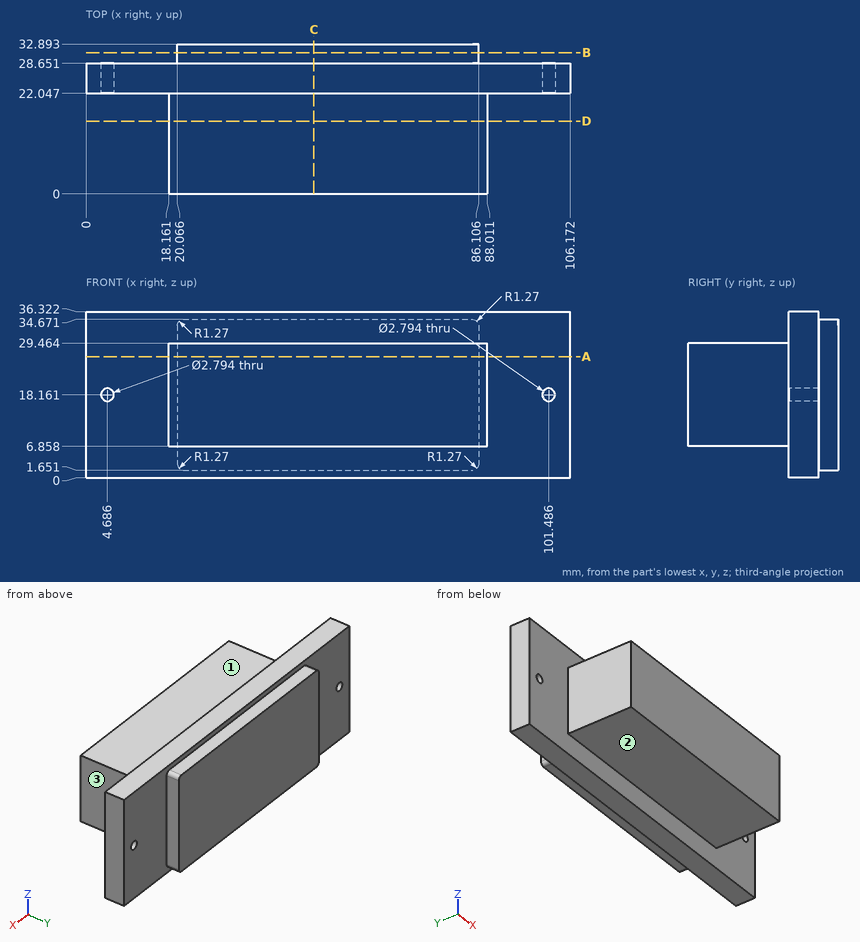
Design review of the part shown in the three views and the two pictorial views. Dimensions are in mm from the part's minimum x, y and z. A direction names the side the tool comes from. Round coordinates to 2 decimals unless told otherwise and drop trailing zeros. Loops run counter-clockwise (first coordinate to the right, second up) from the corner with the lowest first, then second, coordinate; pieces in that order, holes last. Notation, with made-up numbers: (45, 51) -> (58, 51) arc R30 ccw to (58, 90) -> close; hole circle Ø2 at (3.5, -17). An arc over 180 degrees is marked (long way). Answer as a JSON object with one key per item and string values. Group by question number.
1) We need section B-B on y = 31. Write out the cut boundary in (x, z).
2) We need section D-D on y = 16. Write out the cut boundary in (x, z), then the cut area to 3 significant figures.
3) For pin 1 Ø11 at (y, z) = (14, 15) entering from -X; pin 2 Ø6 at (x, y) = (73.5, 16.5) entering from -Z; pin 3 Ø1.3 at (x, y) = (55, 30.5) entering from -Z; pin 4 Ø1.7 at (x, z) = (4.69, 18.16) entering from -Y, all flat-tipped, find the tip position at first contact; note any pin that passes through.
4) For line 1 (X direction, y = 17, z = 22); line 2 (Z direction, x = 27, y = 31.5); line 3 (Y direction, x = 64.5, z = 33.5), list the stretches that pass through material, from the lowest coordinate up. Write a range as [from, to].
5) For the marked faces 1, 2 and 3, list the 3-axis set-ups (+Z, -Z, +X, -X, +Y, -Y) from which the entire face can be reached by the end or side of a thin tool; tool diameter is ignored.
6) We need section A-A on z = 26.5. Write out the cut boundary in (x, y), then the cut area to 3 significant figures.
7) We need section C-C on x = 50. Write out the cut boundary in (y, z), then the cut area to 3 significant figures.
Result set:
{
 "1": {"outline": "(20.07, 2.92) arc R1.27 ccw to (21.34, 1.65) -> (84.84, 1.65) arc R1.27 ccw to (86.11, 2.92) -> (86.11, 33.4) arc R1.27 ccw to (84.84, 34.67) -> (21.34, 34.67) arc R1.27 ccw to (20.07, 33.4) -> close"},
 "2": {"outline": "(18.16, 6.86) -> (88.01, 6.86) -> (88.01, 29.46) -> (18.16, 29.46) -> close", "area": "1,580 mm²"},
 "3": {"pin 1": "x = 18.16", "pin 2": "z = 6.86", "pin 3": "z = 1.65", "pin 4": "through"},
 "4": {"line 1": "[18.16, 88.01]", "line 2": "[1.65, 34.67]", "line 3": "[22.05, 32.89]"},
 "5": {"face 1": "+Z, +X, -X, -Y", "face 2": "-Z, +X, -X, -Y", "face 3": "+Z, -Z, +X, -Y"},
 "6": {"outline": "(0, 22.05) -> (18.16, 22.05) -> (18.16, 0) -> (88.01, 0) -> (88.01, 22.05) -> (106.17, 22.05) -> (106.17, 28.65) -> (86.11, 28.65) -> (86.11, 32.89) -> (20.07, 32.89) -> (20.07, 28.65) -> (0, 28.65) -> close", "area": "2,520 mm²"},
 "7": {"outline": "(0, 6.86) -> (22.05, 6.86) -> (22.05, 0) -> (28.65, 0) -> (28.65, 1.65) -> (32.89, 1.65) -> (32.89, 34.67) -> (28.65, 34.67) -> (28.65, 36.32) -> (22.05, 36.32) -> (22.05, 29.46) -> (0, 29.46) -> close", "area": "878 mm²"}
}
